Autodesk Inventor part; units mm, degrees
ref_plane "YZ Plane" through (0, 0, 0) normal (1, 0, 0) x (0, 1, 0)
ref_plane "XZ Plane" through (0, 0, 0) normal (0, 1, 0) x (-1, 0, 0)
ref_plane "XY Plane" through (0, 0, 0) normal (0, 0, 1) x (1, 0, 0)
sketch "Sketch1" plane through (0, 0, 0) normal (0, 1, 0) x (-1, 0, 0)
  line L0 (45.8955, 52.7129) -> (-54.1045, 52.7129)
  line L1 (-64.1045, 42.7129) -> (-64.1045, -32.2871)
  line L2 (-54.1045, -42.2871) -> (45.8955, -42.2871)
  line L3 (55.8955, -32.2871) -> (55.8955, 42.7129)
  arc A0 (-64.1045, -32.2871) -> (-54.1045, -42.2871) centre (-54.1045, -32.2871) ccw
  arc A1 (-54.1045, 52.7129) -> (-64.1045, 42.7129) centre (-54.1045, 42.7129) ccw
  arc A2 (55.8955, 42.7129) -> (45.8955, 52.7129) centre (45.8955, 42.7129) ccw
  arc A3 (45.8955, -42.2871) -> (55.8955, -32.2871) centre (45.8955, -32.2871) ccw
  point P0 (0, 0)
  dimension "d0" = 120
  dimension "d1" = 95
  dimension "d4" = 10
extrude "Extrusion2" add sketch "Sketch1" along normal blind 3
sketch "Sketch3" plane through (0, 3, 0) normal (0, 1, 0) x (1, 0, 0)
  line L0 (-40.8955, -28.7129) -> (-8.6955, -28.7129)
  line L1 (-8.6955, -28.7129) -> (-8.6955, -25.7129)
  line L2 (-8.6955, -25.7129) -> (-40.8955, -25.7129)
  line L3 (-40.8955, -25.7129) -> (-40.8955, -28.7129)
  line L4 (-40.8955, 15.2871) -> (-8.6955, 15.2871)
  line L5 (-8.6955, 15.2871) -> (-8.6955, 18.2871)
  line L6 (-8.6955, 18.2871) -> (-40.8955, 18.2871)
  line L7 (-40.8955, 18.2871) -> (-40.8955, 15.2871)
  line L8 (-29.7955, -28.7129) -> (-19.7955, -28.7129)
  line L9 (-19.7955, -28.7129) -> (-19.7955, -25.7129)
  line L10 (-19.7955, -25.7129) -> (-29.7955, -25.7129)
  line L11 (-29.7955, -25.7129) -> (-29.7955, -28.7129)
  line L12 (-29.7955, 15.2871) -> (-19.7955, 15.2871)
  line L13 (-19.7955, 15.2871) -> (-19.7955, 18.2871)
  line L14 (-19.7955, 18.2871) -> (-29.7955, 18.2871)
  line L15 (-29.7955, 18.2871) -> (-29.7955, 15.2871)
  line L16 (-55.8955, 32.2871) -> (-55.8955, -42.7129)
  line L17 (-45.8955, -52.7129) -> (54.1045, -52.7129)
  line L18 (54.1045, 42.2871) -> (-45.8955, 42.2871)
  point P0 (0, 0)
  point P1 (-8.6955, -27.2129)
  point P2 (-8.6955, 16.7871)
  dimension "d7" = 32.2
  dimension "d8" = 3
  dimension "d9" = 32.2
  dimension "d10" = 3
  dimension "d11" = 41
  dimension "d12" = 10
  dimension "d13" = 11.1
  dimension "d14" = 10
  dimension "d15" = 11.1
  dimension "d16" = 15
  dimension "d17" = 24
  dimension "d18" = 95
  dimension "d19" = 24
extrude "Extrusion3" cut sketch "Sketch3" against normal blind 10 contours L3 L2 L11 L0 | L9 L2 L1 L0 | L7 L6 L15 L4 | L13 L6 L5 L4
properties part number "Boden"
Source: CAD feature listing. Evaluate the final solid. Frame: model axes, mm. A direction names the side the tool comes from. Coordinates: 2 decimals unless noted, no trailing zeros. Loops run counter-clockwise (first coordinate to the right, second up) from the corner with the lowest first, then second, coordinate; pieces in that order, holes last. Notation, with made-up numbers: (8, 18.5) - (58, 18.5) arc R19 ccw to (58, 22.5) - close; hole circle Ø7 at (66.5, -16.5). An arc over 180 degrees is marked (long way). Answer as CSV lines item,"result".
1. Section A-A (x = -39). Return loops of the section in (y, z), then the cut area to 3 significant figures.
Established:
outline,"(0, -42.29) - (3, -42.29) - (3, -18.29) - (0, -18.29) - close; (0, -15.29) - (3, -15.29) - (3, 25.71) - (0, 25.71) - close; (0, 28.71) - (3, 28.71) - (3, 52.71) - (0, 52.71) - close"
area,"267 mm2"
2. Mould query, pull axis X, two halves, no side actions, for faces 3 (the cylindrical face through (-53.044, 1.479, -39.28)), 4 (the flat face through (5, 1, -42.287)), 5 (the flat face through (-14, 2, 28.713)). Classes: released by +X, released by -X, zero draft, split by the parting line, or undercut.
Established:
face 3,"released by -X"
face 4,"zero draft"
face 5,"undercut"
3. Section B-B (z = 27). Return loops of the section in (x, y).
Established:
outline,"(-55.9, 0) - (-40.9, 0) - (-40.9, 3) - (-55.9, 3) - close; (-29.8, 0) - (-19.8, 0) - (-19.8, 3) - (-29.8, 3) - close; (-8.7, 0) - (64.1, 0) - (64.1, 3) - (-8.7, 3) - close"
4. Reachability of faces 1 (the flat face through (-14, 2, -18.287)), 2 (the flat face through (-55.896, 1, 5)) from +Z, -Z, +X, -X, +Y, -Y: full face, straight path, thin tool, end or side. Return the list, or none.
Established:
face 1,"+Y, -Y"
face 2,"+Z, -Z, -X, +Y, -Y"
5. Section C-C (y = 1.05). Return loops of the section in (x, z).
Established:
outline,"(-55.9, -32.29) arc R10 ccw to (-45.9, -42.29) - (54.1, -42.29) arc R10 ccw to (64.1, -32.29) - (64.1, 42.71) arc R10 ccw to (54.1, 52.71) - (-45.9, 52.71) arc R10 ccw to (-55.9, 42.71) - close; hole (-40.9, -18.29) - (-29.8, -18.29) - (-29.8, -15.29) - (-40.9, -15.29) - close; hole (-40.9, 25.71) - (-29.8, 25.71) - (-29.8, 28.71) - (-40.9, 28.71) - close; hole (-19.8, -18.29) - (-8.7, -18.29) - (-8.7, -15.29) - (-19.8, -15.29) - close; hole (-19.8, 25.71) - (-8.7, 25.71) - (-8.7, 28.71) - (-19.8, 28.71) - close"
6. Ray query, line 1 (Z direction, x = -9.5, y = 1.25); line 2 (X direction, y = 1.3, z = 26.5); line 3 (X direction, y = 1.05, z = 48.5). Return the intervals inside material, ascending.
Established:
line 1,"z = -42.29 to -18.29, -15.29 to 25.71, 28.71 to 52.71"
line 2,"x = -55.9 to -40.9, -29.8 to -19.8, -8.7 to 64.1"
line 3,"x = -54.05 to 62.26"
